from build123d import *

# Parameters (mm, degrees)
F0_R     = 2.5
F0_R_2   = 1.5
F1_DEPTH = 1.5
F2_W     = 6
F2_H     = 3.25
F2_W_2   = 16.5
F2_H_2   = 10.75
F2_H_3   = 13.05
F3_DEPTH = 13
F2_W_3   = 7.5
F2_H_4   = 6
F4_DEPTH = 3
F5_W     = 15
F5_H     = 15
F6_DEPTH = 1.85


with BuildPart() as f1:
    # F0 (on Top) → F1 (new body)
    with BuildSketch(Plane.XY):
        with BuildLine():
            ThreePointArc((0, 1.5875), (0.464968, 0.464968), (1.5875, 0))
            Line((1.5875, 0), (44.7675, 0))
            ThreePointArc((44.7675, 0), (45.890032, 0.464968), (46.355, 1.5875))
            Line((46.355, 1.5875), (46.355, 46.6725))
            ThreePointArc((46.355, 46.6725), (45.890032, 47.795032), (44.7675, 48.26))
            Line((44.7675, 48.26), (1.5875, 48.26))
            ThreePointArc((1.5875, 48.26), (0.464968, 47.795032), (0, 46.6725))
            Line((0, 46.6725), (0, 1.5875))
        make_face()
        with Locations((3.0525, 2.88)):
            Circle(F0_R, mode=Mode.SUBTRACT)
        with Locations((43.3025, 2.88)):
            Circle(F0_R, mode=Mode.SUBTRACT)
        with Locations((3.0525, 45.38)):
            Circle(F0_R, mode=Mode.SUBTRACT)
        with Locations((43.3025, 45.38)):
            Circle(F0_R, mode=Mode.SUBTRACT)
        with Locations((3.0525, 2.88)):
            Circle(F0_R)
        with Locations((3.0525, 2.88)):
            Circle(F0_R_2, mode=Mode.SUBTRACT)
        with Locations((43.3025, 2.88)):
            Circle(F0_R)
        with Locations((43.3025, 2.88)):
            Circle(F0_R_2, mode=Mode.SUBTRACT)
        with Locations((43.3025, 45.38)):
            Circle(F0_R)
        with Locations((43.3025, 45.38)):
            Circle(F0_R_2, mode=Mode.SUBTRACT)
        with Locations((3.0525, 45.38)):
            Circle(F0_R)
        with Locations((3.0525, 45.38)):
            Circle(F0_R_2, mode=Mode.SUBTRACT)
    extrude(amount=F1_DEPTH)

    # F2 (on face) → F3 (join)
    with BuildSketch(Plane.XY.offset(1.5)):
        with Locations((9.5525, 49.885)):
            Rectangle(F2_W, F2_H)
        with Locations((23.5525, 49.885)):
            Rectangle(F2_W_2, F2_H)
        with Locations((9.5525, 42.885)):
            Rectangle(F2_W, F2_H_2)
        with Locations((23.5525, 41.735)):
            Rectangle(F2_W_2, F2_H_3)
    extrude(amount=F3_DEPTH)

    # F2 (on face) → F4 (join)
    with BuildSketch(Plane.XY.offset(1.5)):
        with Locations((10.3025, 3)):
            Rectangle(F2_W_3, F2_H_4)
    extrude(amount=F4_DEPTH)

    # F5 (on face) → F6 (join)
    with BuildSketch(Plane(origin=(0, 0, 0), x_dir=(1, 0, 0), z_dir=(0, 0, -1))):
        with Locations((27.3025, -5)):
            Rectangle(F5_W, F5_H)
    extrude(amount=F6_DEPTH)


solid = f1.part
Model file for the job. Use its own axes, mm. A direction names the side the tool comes from. Give positions to 0.01 mm unless a question says otherwise; leave off trailing zeros. Write each loop counter-clockwise with the first axis right and the second up, starting at its lowest first coordinate (ties: lowest second). Pieces come first, ordered by that corner, then holes. Notation, with made-up numbers: (34.25, 65) -> (48.25, 65) arc R14 cw to (48.25, 75) -> close; hole circle Ø9 at (71, 61.25). An arc over 180 degrees is marked (long way). Write item = value, one per line.
(1) Slice it at D-D, the plane y = 39. Give the cut face in (x, z) (1 decimal), then the cut area to 3 significant figures.
Determined:
outline = (0, 0) -> (46.4, 0) -> (46.4, 1.5) -> (31.8, 1.5) -> (31.8, 14.5) -> (15.3, 14.5) -> (15.3, 1.5) -> (12.6, 1.5) -> (12.6, 14.5) -> (6.6, 14.5) -> (6.6, 1.5) -> (0, 1.5) -> close
area = 362 mm2
(2) Slice it at B-B, the plane y = 2.88. Give the number of separate pieces and of enclosed holes in the cut face, then the cut area to 3 significant figures.
Determined:
separate_pieces = 3
enclosed_holes = 0
area = 111 mm2
(3) Probe line 1 along Z through (x, y) = (15, 23); line 2 along Y through (x, z) = (17, 8.5); line 3 along Y through (x, z) = (7, 12.25). List the from-to ranges inside material, lowest first.
Determined:
line_1 = 0 to 1.5
line_2 = 35.21 to 51.51
line_3 = 37.51 to 51.51
(4) Mould opens along Y. For faces 1 (the face through (45.878, 0.453, 0.74)), 2 (the face through (0.48, 47.81, 0.74)), 3 (the face through (1.86, 1.97, 0.74)) say: released by +Y, released by -Y, zero draft, split by the parting line, or undercut.
Determined:
face_1 = released by -Y
face_2 = released by +Y
face_3 = undercut
(5) Flat gauge pins, fed straight in: P1, Ø3, axis at x = 8.5, z = 11, coming from the -Y side; P2, Ø1, axis at x = 27, y = 37.5, coming from the -Z side; P3, Ø10, axis at x = 40, y = 33.5, coming from the +Z side; P4, Ø4, axis at y = 24.5, z = 4, coming from the -X side. Where does each tip first touch, or does it go through?
Determined:
P1 = 37.51
P2 = 0
P3 = 1.5
P4 = through
(6) Slice it at A-A, the plane z = 5.25. Give the cut face in (x, y).
Determined:
outline = (6.55, 37.51) -> (12.55, 37.51) -> (12.55, 51.51) -> (6.55, 51.51) -> close; (15.3, 35.21) -> (31.8, 35.21) -> (31.8, 51.51) -> (15.3, 51.51) -> close
(7) Tool access for faces 4 (the face through (6.552, 3, 3)), 5 (the face through (23, 48.26, 1)), 6 (the face through (10, 37.51, 8)): list every direction of +Z, -Z, +X, -X, +Y, -Y with a clear straight run to the whole face (end or side of a thin tool).
Determined:
face_4 = +Z, -X, +Y, -Y
face_5 = -Z, +X, -X, +Y
face_6 = +Z, -X
(8) Slice it at C-C, the plane x = 9. Give the cut face in (y, z).
Determined:
outline = (0, 0) -> (48.26, 0) -> (48.26, 1.5) -> (51.51, 1.5) -> (51.51, 14.5) -> (37.51, 14.5) -> (37.51, 1.5) -> (6, 1.5) -> (6, 4.5) -> (0, 4.5) -> close
